```python
from build123d import *

# Parameters (mm, degrees)
SKETCH017_W   = 75
SKETCH017_H   = 95
PAD013_DEPTH  = 3
SKETCH018_W   = 75
SKETCH018_H   = 95
SKETCH018_W_2 = 72.6
SKETCH018_H_2 = 30.066667
SKETCH018_H_3 = 30.066666
SKETCH018_W_3 = 72.757653
PAD014_DEPTH  = 35
FILLET012_R   = 1.8
FILLET013_R   = 10


with BuildPart() as part:
    # Sketch017 → Pad013 (new body)
    with BuildSketch(Plane.XZ):
        Rectangle(SKETCH017_W, SKETCH017_H)
    extrude(amount=PAD013_DEPTH)

    # Sketch018 → Pad014 (join)
    with BuildSketch(Plane.XZ.offset(1)):
        Rectangle(SKETCH018_W, SKETCH018_H)
        with Locations((0, 31.266666)):
            Rectangle(SKETCH018_W_2, SKETCH018_H_2, mode=Mode.SUBTRACT)
        Rectangle(SKETCH018_W_2, SKETCH018_H_3, mode=Mode.SUBTRACT)
        with Locations((-0.078827, -31.266666)):
            Rectangle(SKETCH018_W_3, SKETCH018_H_2, mode=Mode.SUBTRACT)
    extrude(amount=PAD014_DEPTH)

    # Fillet012
    fillet012_edges = [part.edges().sort_by_distance(p)[0] for p in [
        (0, 0, 47.5),
        (37.5, 0, 0),
        (0, 0, -47.5),
        (-37.5, 0, 0),
    ]]
    fillet(fillet012_edges, radius=FILLET012_R)

    # Fillet013
    fillet013_edges = [part.edges().sort_by_distance(p)[0] for p in [
        (36.3, -3, 31.266667),
        (36.3, -3, 0),
        (36.3, -3, -31.266667),
        (-36.3, -3, 31.266667),
        (-36.3, -3, 0),
        (-36.457653, -3, -31.266667),
    ]]
    fillet(fillet013_edges, radius=FILLET013_R)


solid = part.part
```
The listing builds one solid part. Answer for the finished solid, in the listing's coordinates (mm). A direction names the side the tool comes from. Coordinates: 2 decimals unless noted, no trailing zeros. Write each loop counter-clockwise with the first axis right and the second up, starting at its lowest first coordinate (ties: lowest second). Pieces come first, ordered by that corner, then holes. Notation, with made-up numbers: M 87,86 L 98,86 A23 cw 98,111 Z; hole C 6.5,1.5 d9. An arc over 180 degrees is marked long. Use a Markdown table: item, result. Add a question column.
1. Which of the six approach directions +Z, -Z, +X, -X, +Y, -Y give full straight-line access (tool end or side, diameter ignored) to faces 4 (the flat face through (-1, -19, -47.5)), 5 (the flat face through (-1, -19, 16.233))?
2. Straight lines are drawn through the part: line 1 along Z through (x, y) = (-29.5, -32); line 2 along X through (y, z) = (-16.5, -28.5); line 3 along X through (y, z) = (-32.5, 2). For each, find the intervals that lie inside material, in ascending order. Write a range as [from, to].
3. Section C-C (x = -2) is taken. Give the vertices of the cut face in (y, z), plus the area to 3 significant figures.
4. Section A-A (y = -31.5) is taken. Give the vertices of the cut face in (x, z).
5. For a pull along X with two mould halves and no side action, classify faces 1 (the cylindrical face through (-33.45, -6.01, 31.06)), 2 (the flat face through (-1, -19, 47.5)), 3 (the flat face through (-37.5, -19, -1)) as +X half, -X half, draft (parallel to the pull), parting line (faces both ways), or undercut.
6. Given P1, Ø15, axis at x = 0.5, z = -6.5, coming from the -Y side, flat-ended and moving along its own axis, determine where the tip first touches the part or whether it passes through.
7. Section D-D (z = 25) is taken. Give the vertices of the cut face in (x, y).
8. Section B-B (z = -22.5) is taken. Give the vertices of the cut face in (x, y).
Data:
| question | item | result |
|---|---|---|
| 1 | face 4 | -Z, +X, -X, +Y, -Y |
| 1 | face 5 | -Y |
| 2 | line 1 | z = [-47.5, -46.3], [-16.23, -15.03], [15.03, 16.23], [46.3, 47.5] |
| 2 | line 2 | x = [-37.5, -36.46], [36.3, 37.5] |
| 2 | line 3 | x = [-37.5, -36.3], [36.3, 37.5] |
| 3 | outline | M -36,-47.5 L -1.8,-47.5 A1.8 ccw 0,-45.7 L 0,45.7 A1.8 ccw -1.8,47.5 L -36,47.5 L -36,46.3 L -3,46.3 L -3,16.23 L -36,16.23 L -36,15.03 L -3,15.03 L -3,-15.03 L -36,-15.03 L -36,-16.23 L -3,-16.23 L -3,-46.3 L -36,-46.3 Z |
| 3 | area | 442 mm2 |
| 4 | outline | M -37.5,-47.5 L 37.5,-47.5 L 37.5,47.5 L -37.5,47.5 Z; hole M -36.46,-46.3 L 36.3,-46.3 L 36.3,-16.23 L -36.46,-16.23 Z; hole M -36.3,-15.03 L 36.3,-15.03 L 36.3,15.03 L -36.3,15.03 Z; hole M -36.3,16.23 L 36.3,16.23 L 36.3,46.3 L -36.3,46.3 Z |
| 5 | face 1 | undercut |
| 5 | face 2 | draft |
| 5 | face 3 | -X half |
| 6 | P1 | stops at y = -3 |
| 7 | outline | M -37.5,-36 L -36.3,-36 L -36.3,-13 A10 cw -26.3,-3 L 26.3,-3 A10 cw 36.3,-13 L 36.3,-36 L 37.5,-36 L 37.5,-1.8 A1.8 ccw 35.7,0 L -35.7,0 A1.8 ccw -37.5,-1.8 Z |
| 8 | outline | M -37.5,-36 L -36.46,-36 L -36.46,-13 A10 cw -26.46,-3 L 26.3,-3 A10 cw 36.3,-13 L 36.3,-36 L 37.5,-36 L 37.5,-1.8 A1.8 ccw 35.7,0 L -35.7,0 A1.8 ccw -37.5,-1.8 Z |
